Autodesk Inventor part; units mm, degrees
ref_plane "YZ Plane" through (0, 0, 0) normal (1, 0, 0) x (0, 1, 0)
ref_plane "XZ Plane" through (0, 0, 0) normal (0, 1, 0) x (-1, 0, 0)
ref_plane "XY Plane" through (0, 0, 0) normal (0, 0, 1) x (1, 0, 0)
sketch "Sketch1" plane through (0, 0, 0) normal (0, 0, 1) x (1, 0, 0)
  line L0 (15, -7) -> (-15, -7)
  line L1 (-15, -7) -> (-15, 7)
  line L2 (-15, 7) -> (15, 7)
  line L3 (15, 7) -> (15, -7)
  line L4 (15, -7) -> (-15, 7) construction
  line L5 (-15, -7) -> (15, 7) construction
  point P0 (0, 0)
  dimension "d0" = 30
  dimension "d1" = 14
extrude "Extrusion1" add sketch "Sketch1" along normal blind 30
sketch "Sketch3" plane through (15, -7, 0) normal (1, 0, 0) x (0, 0, -1)
  line L0 (0, 0) -> (-30, 0)
  line L1 (-15, 0) -> (-15, -2)
  arc A0 (-5.7129, 0) -> (-24.2871, 0) centre (-15, -2) ccw
  point P0 (0, 7)
  dimension "d4" = 2
  dimension "d5" = 19
extrude "Extrusion2" cut sketch "Sketch3" against normal blind 25
sketch "Sketch5" plane through (-15, 7, 0) normal (0, 1, 0) x (1, 0, 0)
  line L0 (30, 0) -> (0, 0)
  line L1 (30, -30) -> (0, -30)
  line L2 (0, -30) -> (0, -27.25)
  line L3 (0, 0) -> (0, -30)
  line L4 (0, -27.25) -> (2.75, -27.25)
  circle A0 centre (2.75, -27.25) radius 2
  line L5 (0, 0) -> (0, -2.75)
  line L6 (0, -2.75) -> (2.75, -2.75)
  circle A1 centre (2.75, -2.75) radius 2
  line L7 (2.75, -27.25) -> (10.75, -27.25)
  circle A2 centre (10.75, -27.25) radius 1.5875
  point P0 (15, 0)
  dimension "d11" = 2.75
  dimension "d12" = 2.75
  dimension "d13" = 4
  dimension "d14" = 2.75
  dimension "d15" = 2.75
  dimension "d16" = 4
  dimension "d17" = 8
  dimension "d18" = 3.175
extrude "Extrusion3" cut sketch "Sketch5" against normal blind 100 contours A2
sketch "Sketch6" plane through (-15, 7, 0) normal (0, 1, 0) x (1, 0, 0)
  point P0 (15, 0)
sketch "Sketch7" plane through (15, -7, 0) normal (1, 0, 0) x (0, 0, -1)
  line L0 (0, 14) -> (-30, 14)
  line L1 (-30, 14) -> (-25, 14)
  line L2 (-25, 14) -> (-25, 9)
  line L3 (0, 14) -> (0, 0)
  line L4 (0, 14) -> (-5, 14)
  line L5 (-5, 14) -> (-5, 9)
  circle A0 centre (-25, 9) radius 3
  circle A1 centre (-5, 9) radius 3
  point P0 (0, 7)
  dimension "d21" = 5
  dimension "d22" = 5
  dimension "d23" = 5
  dimension "d24" = 5
  dimension "d25" = 6
  dimension "d26" = 6
extrude "Extrusion4" cut sketch "Sketch7" against normal blind 15
move or copy body "Move Body1" bodies to move or copy 1 copy no translate (-20, 0, 0)
move or copy body "Move Body2" bodies to move or copy 1 copy no translate (-5, 0, 0)
sketch "Sketch8" plane through (0, 0, 0) normal (1, 0, 0) x (0, 1, 0)
  point P0 (0, 0)
sketch "Sketch9" plane through (-40, 7, 0) normal (0, 1, 0) x (1, 0, 0)
  line L0 (30, -30) -> (0, -30)
  line L1 (0, -30) -> (0, -27.25)
  line L2 (0, 0) -> (0, -30)
  line L3 (0, -27.25) -> (3, -27.25)
  circle A0 centre (3, -27.25) radius 2
  line L4 (0, 0) -> (0, -2.75)
  line L5 (0, -2.75) -> (3, -2.75)
  circle A1 centre (3, -2.75) radius 2
  point P0 (40, 0)
  dimension "d35" = 2.75
  dimension "d36" = 3
  dimension "d37" = 4
  dimension "d38" = 2.75
  dimension "d39" = 4
  dimension "d40" = 3
extrude "Extrusion5" cut sketch "Sketch9" against normal blind 14
sketch "Sketch14" plane through (-40, 7, 30) normal (0, 0, 1) x (1, 0, 0)
  line L0 (30, 0) -> (0, 0)
  line L1 (30, 0) -> (25, 0)
  line L2 (25, 0) -> (25, -5)
  circle A0 centre (25, -5) radius 2
  point P0 (40, -7)
  dimension "d47" = 5
  dimension "d48" = 5
  dimension "d49" = 4
extrude "Extrusion6" cut sketch "Sketch14" against normal blind 3
sketch "Sketch15" plane through (-10, 7, 0) normal (0, 0, -1) x (-1, 0, 0)
  line L0 (0, -14) -> (0, 0)
  line L1 (0, 0) -> (5, 0)
  line L2 (0, 0) -> (30, 0)
  line L3 (5, 0) -> (5, -5)
  circle A0 centre (5, -5) radius 2
  point P0 (-10, -7)
  dimension "d52" = 5
  dimension "d53" = 5
  dimension "d54" = 4
extrude "Extrusion7" cut sketch "Sketch15" against normal blind 4
thread "Thread3"
thread "Thread4"
sketch "Sketch16" plane through (-40, -7, 0) normal (-1, 0, 0) x (0, 0, 1)
  line L0 (0, 14) -> (30, 14)
  line L1 (0, 14) -> (15, 14)
  line L2 (15, 14) -> (15, -2)
  circle A0 centre (15, -2) radius 7.5
  point P0 (0, 7)
  dimension "d61" = 16
  dimension "d62" = 15
extrude "Extrusion8" cut sketch "Sketch16" against normal blind 15
move or copy body "Move Body3" bodies to move or copy 1 copy no translate (25, 0, 0)
move or copy body "Move Body4" bodies to move or copy 1 copy no translate (10, 0, -15)
move or copy body "Move Body5" bodies to move or copy 1 copy no translate (-10, 0, 0)
equation "\"d55\" = d54"
properties part number "Rb oven housing top-back" material "Copper"
The model under review builds one solid part; all positions refer to its coordinate system, in mm. A direction names the side the tool comes from. Coordinates: 2 decimals unless noted, no trailing zeros. Order: outer loops, then holes, each group sorted by start corner. A loop starts at its lowest first (then second) coordinate and runs counter-clockwise, first axis right, second up. Notation, with made-up numbers: (-18, 76) -> (28, 76) arc R17 cw to (28, 86) -> close; hole circle Ø4 at (-14, 50). An arc over 180 degrees is marked (long way). Answer in a Markdown table with one row per item. Add a question column.
Item 1: We need section C-C on x = 10. Write out the cut boundary in (y, z), plus the area to 3 significant figures.
Item 2: We need section A-A on y = 2. Give the number of separate pieces and of enclosed holes in the cut face, plus the area to 3 significant figures.
Item 3: Mouldability with a two-part tool opening along Z and no side actions: class faces 4 (the flat face through (0, 0, -15)), 5 (the flat face through (15, 2, 0)), 6 (the flat face through (0, 0, 15)), 7 (the cylindrical face through (7.6, 2.9, 7.14)) as +Z half, -Z half, draft (parallel to the pull), parting line (faces both ways), or undercut.
Item 4: Machinability: for faces 1 (the flat face through (0, 2, -10)), 2 (the cylindrical face through (11.474, 3.352, -13.944)), 3 (the flat face through (-10, -1, 0)), which of the approach directions +Z, -Z, +X, -X, +Y, -Y give a long, thin tool a straight path to every point of the face, cutting with its end or side? Answer none if there is none.
Item 5: To check wall thickness, follow probe 1 along X at (y, z) = (3, 12.25); probe 2 along Z at (x, y) = (-12, -0.5); probe 3 along X at (y, z) = (-0.5, 12.25). State the ranges of each line that lie inside material, in increasing order.
Item 6: Clearance check with a flat-ended pin moving along its axis: pin 1 (1.8 mm diameter, centred on y = 1.5, z = 9.5, fed in from +X). State where the tip first meets the part, or that it passes through.
Final values:
| question | item | result |
|---|---|---|
| 1 | outline | (-7, -15) -> (0, -15) -> (0, -12.24) arc R3 cw (long way) to (4, -12.24) -> (4, -15) -> (7, -15) -> (7, 15) -> (4, 15) -> (4, 12.24) arc R3 cw (long way) to (0, 12.24) -> (0, 15) -> (-7, 15) -> (-7, 9.29) arc R9.5 cw to (-7, -9.29) -> close |
| 1 | area | 241 mm2 |
| 2 | separate pieces | 3 |
| 2 | enclosed holes | 3 |
| 2 | area | 671 mm2 |
| 3 | face 4 | -Z half |
| 3 | face 5 | draft |
| 3 | face 6 | +Z half |
| 3 | face 7 | undercut |
| 4 | face 1 | +X |
| 4 | face 2 | -Z |
| 4 | face 3 | +X, -Y |
| 5 | probe 1 | x = -15 to -14, -10 to -5.84, -2.66 to 0 |
| 5 | probe 2 | z = -15 to -14.25, -10.25 to 10.25, 14.25 to 15 |
| 5 | probe 3 | x = -15 to -14, -10 to -5.84, -2.66 to 15 |
| 6 | pin 1 | stops at x = 0 |
